Input: part model. Units: mm. Frame: model coordinates. A direction names the side the tool comes from. Round coordinates to 2 decimals unless told otherwise and drop trailing zeros. Loops run counter-clockwise (first coordinate to the right, second up) from the corner with the lowest first, then second, coordinate; pieces in that order, holes last.
(1) Access query for faces 1 (the face through (12.84, -54.73, 21.03)), 2 (the face through (14, -53.7, 25.5)). Directions: +Z, -Z, +X, -X, +Y, -Y. A direction counts if a zero-diameter tool reaches every point of the face in a straight line with its end or side. Return the directions, or none.
(2) Cut plane A-A, the plane y = -50. Output: boundary loops of the cut face in (x, z), and give its area (4 significant figures).
(3) Line query: line 1 (Z direction, x = 22.25, y = -44.75); line 2 (Y direction, x = 12, z = 22.5); line 3 (X direction, y = -54, z = 26.5). Output: solid intervals per line, ascending.
(4) Cut plane B-B, the plane x = 18. Output: boundary loops of the cut face in (y, z).
(5) First-contact query: pin 1 Ø2 at (x, z) = (23, 20.5) entering from +Y; pin 2 Ø5 at (x, z) = (14.5, 20) entering from +Y. Flat tips, straight axial feed; report the tip coordinate or a pass-through.
(6) Cut plane C-C, the plane z = 21.75. Output: boundary loops of the cut face in (x, y).
from build123d import *

# Parameters (mm, degrees)
CYLINDER001_R            = 7
CYLINDER001_DEPTH        = 4
CYLINDER_R               = 5.45
CYLINDER_DEPTH           = 5
CLONE018_PLACEMENT_ANGLE = 180


with BuildPart() as knob002:
    # Cylinder001 → Cylinder001 (new body)
    with BuildSketch(Plane(origin=(7, 0, -5), x_dir=(1, 0, 0), z_dir=(0, 0, 1))):
        Circle(CYLINDER001_R)
    extrude(amount=CYLINDER001_DEPTH)


with BuildPart() as knob004:
    # Cylinder → Cylinder (new body)
    with BuildSketch(Plane(origin=(7, 0, -10), x_dir=(1, 0, 0), z_dir=(0, 0, 1))):
        Circle(CYLINDER_R)
    extrude(amount=CYLINDER_DEPTH)

    # Fusion007: union knob002
    add(knob002.part)


with BuildPart() as knob004_1:
    # Clone018 placement: moved
    add(knob004.part.moved(Location((11, -50, 18))).rotate(Axis((11, -50, 18), (1, 0, 0)), CLONE018_PLACEMENT_ANGLE))


solid = knob004_1.part
Reported:
1. face 1: +Z, -Z
1. face 2: +Z
2. outline: (11, 19) - (25, 19) - (25, 23) - (23.45, 23) - (23.45, 28) - (12.55, 28) - (12.55, 23) - (11, 23) - close
2. area: 110.5 mm2
3. line 1: z = 19 to 23
3. line 2: y = -53.61 to -46.39
3. line 3: x = 14.3 to 21.7
4. outline: (-57, 19) - (-43, 19) - (-43, 23) - (-44.55, 23) - (-44.55, 28) - (-55.45, 28) - (-55.45, 23) - (-57, 23) - close
5. pin 1: stops at y = -44.26
5. pin 2: stops at y = -43.07
6. outline: circle Ø14 at (18, -50)
